```python
from build123d import *

# Parameters (mm, degrees)
PAD_DEPTH       = 15
POCKET_DEPTH    = 15.001
POCKET001_DEPTH = 15.001
POCKET002_DEPTH = 15.001


with BuildPart() as part:
    # Sketch → Pad (new body)
    with BuildSketch(Plane.XY):
        Polygon((86.032137, 203.51933), (86.032137, 185.207711), (5.370759, 110.416387), (30, 30), (30, 0), (0, 0), (0, 30), (-53.22371, 106.011336), align=None)
    extrude(amount=PAD_DEPTH)

    # Sketch001 (on Face10 of Pad) → Pocket (cut, through all)
    with BuildSketch(Plane.XY.offset(15)):
        Polygon((-32.332783, 102.327701), (-12.257608, 73.65738), (6.170493, 73.65738), (-7.858915, 119.464488), align=None)
    extrude(amount=-POCKET_DEPTH, mode=Mode.SUBTRACT)

    # Sketch002 (on Face5 of Pocket) → Pocket001 (cut, through all)
    with BuildSketch(Plane.XY.offset(15)):
        Polygon((-1.770811, 133.734171), (76.032137, 188.212382), (2.442314, 119.977988), align=None)
    extrude(amount=-POCKET001_DEPTH, mode=Mode.SUBTRACT)

    # Sketch003 (on Face5 of Pocket001) → Pocket002 (cut, through all)
    with BuildSketch(Plane.XY.offset(15)):
        Polygon((-7.930737, 59.294992), (5.340032, 59.294992), (15.657585, 25.607376), align=None)
    extrude(amount=-POCKET002_DEPTH, mode=Mode.SUBTRACT)


solid = part.part
```
Can you work these out from the model? Positions are in its coordinate system, mm. A direction names the side the tool comes from. Give positions to 0.01 mm unless a question says otherwise; leave off trailing zeros. Loops run counter-clockwise (first coordinate to the right, second up) from the corner with the lowest first, then second, coordinate; pieces in that order, holes last. Notation, with made-up numbers: M 1,84 L 13,84 A23 cw 13,120 Z; hole C 28,40 d8. An arc over 180 degrees is marked long. Use one line per item in the form item = value. Start each with the question number.
(1) Thinking about a two-plate mould opening in Y: for faces 4 (the flat face through (-26.239, 67.474, 7.395)), 5 (the flat face through (39.75, 154.57, 7.6)), 6 (the flat face through (86.032, 194, 7)), which applies, released by +Y, released by -Y, zero draft, split by the parting line, or undercut?
(2) I want a section at D-D, the plane x = 12. Write out the boundary of the cut face in (y, z).
(3) I want a section at C-C, the plane x = 32. Write out the boundary of the cut face in (y, z).
(4) On a 3-axis mill with a long thin cutter (end or side, diameter ignored), from which of +Z, -Z, +X, -X, +Y, -Y can I reach the whole of each face in a straight line? I mean faces 1 (the flat face through (30, 15, 7)), 2 (the flat face through (0, 15, 7)), 3 (the flat face through (-0.746, 96.24, 7.605)). Say none if no direction works.
(5) I want a section at B-B, the plane y = 123.5. Write out the boundary of the cut face in (x, z), and give its area (3 significant figures).
(6) I want a section at A-A, the plane z = 8.75. Write out the boundary of the cut face in (x, y) (1 decimal).
(7) Please list where these lines run through material, in increasing order: line 1 (X direction, y = 32.5, z = 1.75); line 2 (Y direction, x = 32.5, z = 13.75); line 3 (X direction, y = 97, z = 4).
(8) I'm going to push flat-ended pins straight in: P1, Ø5, axis at y = 33, z = 12, coming from the -X side; P2, Ø4.5, axis at y = 21, z = 9.5, coming from the +X side; P3, Ø6, axis at y = 130, z = 4, coming from the -X side; P4, Ø8, axis at x = 17.5, z = 6, coming from the -Y side. Where does each tip first touch, or does it pass through?
Worked out:
q1.face_4 = released by -Y
q1.face_5 = undercut
q1.face_6 = zero draft
q2.outline = M 0,0 L 30.83,0 L 30.83,15 L 0,15 Z; M 37.55,0 L 88.77,0 L 88.77,15 L 37.55,15 Z; M 116.56,0 L 128.84,0 L 128.84,15 L 116.56,15 Z; M 143.38,0 L 151.68,0 L 151.68,15 L 143.38,15 Z
q3.outline = M 135.11,0 L 147.38,0 L 147.38,15 L 135.11,15 Z; M 157.38,0 L 165.69,0 L 165.69,15 L 157.38,15 Z
q4.face_1 = +Z, -Z, +X, -Y
q4.face_2 = +Z, -Z, -X, -Y
q4.face_3 = +Z, -Z
q5.outline = M -28.25,0 L 1.36,0 L 1.36,15 L -28.25,15 Z; M 6.24,0 L 19.48,0 L 19.48,15 L 6.24,15 Z
q5.area = 643 mm²
q6.outline = M -53.2,106 L 0,30 L 0,0 L 30,0 L 30,30 L 5.4,110.4 L 86,185.2 L 86,203.5 Z; hole M -32.3,102.3 L -12.3,73.7 L 6.2,73.7 L -7.9,119.5 Z; hole M -7.9,59.3 L 15.7,25.6 L 5.3,59.3 Z; hole M -1.8,133.7 L 2.4,120 L 76,188.2 Z
q7.line_1 = -1.75 to 10.83, 13.55 to 29.23
q7.line_2 = 135.57 to 147.85, 157.73 to 166.04
q7.line_3 = -46.91 to -28.6, -0.98 to 9.48
q8.P1 = -3.85
q8.P2 = 30
q8.P3 = -23.25
q8.P4 = 0
